Verification items for the finished model (mm, model axes). A direction names the side the tool comes from. Give positions to 0.01 mm unless a question says otherwise; leave off trailing zeros. Write each loop counter-clockwise with the first axis right and the second up, starting at its lowest first coordinate (ties: lowest second). Pieces come first, ordered by that corner, then holes. Notation, with made-up numbers: M -16,65.25 L 35,65.25 A22 cw 35,75.25 Z; hole C 60,-3 d2. An arc over 180 degrees is marked long. Write item = value, one per line.
from build123d import *

# Parameters (mm, degrees)
SKETCH1_R               = 25
SKETCH1_R_2             = 8.5
BOSS_EXTRUDE1_DEPTH     = 8
SKETCH2_W               = 16
SKETCH2_H               = 46.314561435
BOSS_EXTRUDE2_DEPTH     = 8
SKETCH3_W               = 16
SKETCH3_H               = 96.314561435
BOSS_EXTRUDE3_DEPTH     = 8
SKETCH4_W               = 16.314561435
SKETCH4_H               = 16
BOSS_EXTRUDE4_DEPTH     = 8
CUT_EXTRUDE1_DEPTH      = 127.743836142
CUT_EXTRUDE1_DEPTH_BACK = 127.743836142
SKETCH5_W               = 48
SKETCH5_H               = 0.5
FILLET1_R               = 5
SKETCH7_W               = 3
SKETCH7_H               = 5.5


with BuildPart() as part:
    # Sketch1 → Boss-Extrude1 (new, symmetric)
    with BuildSketch(Plane.XY):
        Circle(SKETCH1_R)
        Circle(SKETCH1_R_2, mode=Mode.SUBTRACT)
    extrude(amount=BOSS_EXTRUDE1_DEPTH, both=True)

    # Sketch2 → Boss-Extrude2 (add, symmetric)
    with BuildSketch(Plane.XY):
        with Locations((0, 46.842719282)):
            Rectangle(SKETCH2_W, SKETCH2_H)
    extrude(amount=BOSS_EXTRUDE2_DEPTH, both=True)

    # Sketch3 → Boss-Extrude3 (add, symmetric)
    with BuildSketch(Plane.XY):
        with Locations((0, -71.842719283)):
            Rectangle(SKETCH3_W, SKETCH3_H)
    extrude(amount=BOSS_EXTRUDE3_DEPTH, both=True)

    # Sketch4 → Boss-Extrude4 (add, symmetric)
    with BuildSketch(Plane.XY):
        with Locations((31.842719282, 0)):
            Rectangle(SKETCH4_W, SKETCH4_H)
    extrude(amount=BOSS_EXTRUDE4_DEPTH, both=True)

    # Sketch5 → Cut-Extrude1 (cut, two sides: drawn at the far end of the back side and taken through both)
    with BuildSketch(Plane.XY.offset(-CUT_EXTRUDE1_DEPTH_BACK)):
        with Locations((26, 0)):
            Rectangle(SKETCH5_W, SKETCH5_H)
    extrude(amount=CUT_EXTRUDE1_DEPTH + CUT_EXTRUDE1_DEPTH_BACK, mode=Mode.SUBTRACT)

    # Fillet1
    fillet1_edges = [part.edges().sort_by_distance(p)[0] for p in [
        (8, 23.685438565, 0),
        (-8, 23.685438565, 0),
        (8, -23.685438565, 0),
        (-8, -23.685438565, 0),
        (23.685438565, -8, 0),
        (23.685438565, 8, 0),
    ]]
    fillet(fillet1_edges, radius=FILLET1_R)

    # Sketch7 → Cut-Revolve1 (revolve, cut)
    with BuildSketch(Plane(origin=(0, 0, 0), x_dir=(0, 0, -1), z_dir=(1, 0, 0))):
        with Locations((6.5, 11.25)):
            Rectangle(SKETCH7_W, SKETCH7_H)
    revolve(axis=Axis((0, 0, 0), (0, 0, -1)), mode=Mode.SUBTRACT)


solid = part.part
1) Depth check by flat-ended pin: P1, Ø8.5, axis at x = 5.5, y = 3, coming from the -Z side; P2, Ø6, axis at y = 19.5, z = 5, coming from the -X side; P3, Ø8, axis at y = 58.5, z = -1, coming from the +X side. Enter the tip coordinate at first touch or a pass-through.
From the geometry:
P1 = -5
P2 = -18.78
P3 = 8
2) Cross-section at C-C on x = -18.5. Record the boundary of the cut face in (y, z), plus the area to 3 significant figures.
From the geometry:
outline = M -16.82,-8 L 16.82,-8 L 16.82,8 L -16.82,8 Z
area = 538 mm^2
3) Draft check along Y on faces 1 (the cylindrical face through (8.746, 24.409, 0.112)), 2 (the flat face through (33, -8, 0)), 3 (the flat face through (24, 0.25, 0)). Enter one of: +Y half, -Y half, draft (parallel to the pull), parting line (faces both ways), or undercut.
From the geometry:
face_1 = +Y half
face_2 = -Y half
face_3 = undercut
4) Cross-section at A-A on z = 2.75. Record the boundary of the cut face in (x, y).
From the geometry:
outline = M -10.83,-22.53 A5 cw -8,-27.04 L -8,-120 L 8,-120 L 8,-27.04 A5 cw 10.83,-22.53 A25 ccw 22.53,-10.83 A5 cw 27.04,-8 L 40,-8 L 40,-0.25 L 8.5,-0.25 A8.5 cw long 8.5,0.25 L 40,0.25 L 40,8 L 27.04,8 A5 cw 22.53,10.83 A25 ccw 10.83,22.53 A5 cw 8,27.04 L 8,70 L -8,70 L -8,27.04 A5 cw -10.83,22.53 A25 ccw Z
5) Material ranges on probe 1 along Y at (x, z) = (31.5, 1); probe 2 along Y at (x, z) = (0, -7.35); probe 3 along X at (y, z) = (0, -6.25), recorded low to high. Write a range as from..to.
From the geometry:
probe_1 = -8..-0.25, 0.25..8
probe_2 = -120..-14, 14..70
probe_3 = -25..-14
6) Cross-section at B-B on y = -91.5. Record the boundary of the cut face in (x, z), plus the area to 3 significant figures.
From the geometry:
outline = M -8,-8 L 8,-8 L 8,8 L -8,8 Z
area = 256 mm^2
7) Tool access check on faces 4 (the flat face through (24, -0.25, 0)), 5 (the flat face through (8, -74, 0)), 6 (the flat face through (0, -24, 8)), 7 (the flat face through (-8, -74, 0)), 8 (the flat face through (33, 8, 0)). Record the directions out of +Z, -Z, +X, -X, +Y, -Y that give a thin tool (end or side, any length) a straight path to the whole face; none if there is none.
From the geometry:
face_4 = +Z, -Z, +X
face_5 = +Z, -Z, +X, -Y
face_6 = +Z, +X, -X, +Y, -Y
face_7 = +Z, -Z, -X, -Y
face_8 = +Z, -Z, +X, +Y
